Source: CAD feature listing. Evaluate the final solid. Frame: model axes, mm. A direction names the side the tool comes from. Give positions to 0.01 mm unless a question says otherwise; leave off trailing zeros. Write each loop counter-clockwise with the first axis right and the second up, starting at its lowest first coordinate (ties: lowest second). Pieces come first, ordered by that corner, then holes. Notation, with made-up numbers: M -2.75,11 L 14.25,11 A17 ccw 14.25,32 Z; hole C 12,8 d10. An arc over 180 degrees is marked long. Return JSON: item names as keys, results as strings.
Autodesk Inventor part; units mm, degrees
ref_plane "YZ Plane" through (0, 0, 0) normal (1, 0, 0) x (0, 1, 0)
ref_plane "XZ Plane" through (0, 0, 0) normal (0, 1, 0) x (-1, 0, 0)
ref_plane "XY Plane" through (0, 0, 0) normal (0, 0, 1) x (1, 0, 0)
sketch "草图1" plane through (0, 0, 0) normal (0, 1, 0) x (-1, 0, 0)
  line L0 (0, 0) -> (27, 0)
  line L1 (27, 0) -> (27, -44)
  line L2 (27, -44) -> (0, -44)
  line L3 (0, -44) -> (0, 0)
  dimension "d0" = 44
  dimension "d1" = 27
extrude "拉伸1" add sketch "草图1" along normal blind 10
sketch "草图2" plane through (-27, 0, 0) normal (0, 0, 1) x (1, 0, 0)
  line L0 (0, 10) -> (27, 10)
  line L1 (13.5, 10) -> (13.5, 0)
  line L2 (13.5, 10) -> (7.5, 10)
  line L3 (7.5, 10) -> (19.5, 10)
  line L4 (7.5, 10) -> (7.5, 0)
  line L5 (0, 0) -> (27, 0)
  line L6 (19.5, 10) -> (19.5, 0)
  line L7 (7.5, 0) -> (19.5, 0)
  line L8 (7.5, 0) -> (19.5, 0)
  line L9 (19.5, 0) -> (19.5, 8)
  line L10 (19.5, 8) -> (7.5, 8)
  line L11 (7.5, 8) -> (7.5, 0)
  point P0 (7.5, 8)
  dimension "d19" = 6
  dimension "d20" = 12
  dimension "d21" = 8
extrude "拉伸2" cut sketch "草图2" against normal through all contours L10 L1 L5 L4 | L10 L6 L5 L1
sketch "草图3" plane through (-27, 10, 0) normal (0, 0, 1) x (1, 0, 0)
  line L0 (7.5, -10) -> (7.5, -2)
  circle A0 centre (7.5, -6) radius 1.5
  line L1 (19.5, -2) -> (19.5, -10)
  circle A1 centre (19.5, -6) radius 1.5
  point P0 (27, -10)
  point P1 (19.5, -7.5)
  point P2 (19.5, -4.5)
  point P3 (7.5, -4.5)
  point P4 (7.5, -7.5)
  dimension "d22" = 3
  dimension "d23" = 3
extrude "拉伸3" add sketch "草图3" against normal blind 44 contours L0 A0 | L1 A1 picked at (8.2992, -6.2203) picked at (19.2676, -6.4427)
sketch "草图4" plane through (0, 10, 0) normal (0, 1, 0) x (1, 0, 0)
  circle A0 centre (-23, 34) radius 1.5
  line L0 (-6, 44) -> (-21, 44)
  circle A1 centre (-4, 34) radius 1.5
  circle A2 centre (-23, 10) radius 1.5
  circle A3 centre (-4, 10) radius 1.5
  line L1 (-27.606, 22) -> (3.9148, 22)
  line L2 (-13.5, 45.1542) -> (-13.5, -11.9454)
  point P0 (0, 0)
  point P1 (-27, 44)
  dimension "d15" = 3
  dimension "d24" = 12
  dimension "d25" = 9.5
extrude "拉伸4" cut sketch "草图4" against normal blind 10
equation "\"折弯半径\" = 厚度"
equation "\"折弯释压宽度\" = 厚度"
equation "\"折弯释压深度\" = 0.5 * 厚度"
equation "\"拐角释压尺寸\" = 4 * 厚度"
equation "\"最小余量\" = 2 * 厚度"
equation "\"过渡半径\" = 折弯半径"
equation "\"Jacobi半径尺寸\" = 折弯半径"
equation "\"间隙大小\" = 厚度"
properties part number "滑轨座"
1) Draft query along X for faces 4 (the face through (-27, 5, -22)), 5 (the face through (-2.614, 5.07, -9.425)), 6 (the face through (-23.325, 5.07, -32.536)), 7 (the face through (-13.3, 8.3, 0)). Return one class per face: released by +X, released by -X, zero draft, split by the parting line, or undercut.
Numbers:
{"face 4": "released by -X", "face 5": "undercut", "face 6": "undercut", "face 7": "zero draft"}
2) Set-up query: faces 1 (the face through (-18, 4, -22)), 2 (the face through (-24.5, 5.07, -10.07)), 3 (the face through (-7.5, 1, -22)). Return all of +Z, -Z, +X, -X, +Y, -Y with unobstructed straight access to the full face (end or side cutting, diameter ignored); none if empty.
Numbers:
{"face 1": "+Z, -Z", "face 2": "+Y, -Y", "face 3": "+Z, -Z, -Y"}
3) Cut plane A-A, the plane y = 4. Return the cut outline in (x, z), then the cut area to 3 significant figures.
Numbers:
{"outline": "M -27,-44 L -18,-44 L -18,0 L -27,0 Z; M -9,-44 L 0,-44 L 0,0 L -9,0 Z; hole C -23,-34 d3; hole C -23,-10 d3; hole C -4,-34 d3; hole C -4,-10 d3", "area": "764 mm²"}
4) Contact query for flat-ended pins moving along their axis: pin 1 Ø2.5 at (x, z) = (-4, -34) entering from -Y; pin 2 Ø5 at (x, z) = (-15, -37) entering from -Y. Output: stop coordinate, or through.
Numbers:
{"pin 1": "passes through", "pin 2": "stops at y = 8"}
5) Cut plane C-C, the plane z = -10. Return the cut outline in (x, y), then the cut area to 3 significant figures.
Numbers:
{"outline": "M -27,0 L -24.5,0 L -24.5,10 L -27,10 Z; M -21.5,0 L -19.5,0 L -19.5,2.5 A1.5 ccw -19.5,5.5 L -19.5,8 L -7.5,8 L -7.5,5.5 A1.5 ccw -7.5,2.5 L -7.5,0 L -5.5,0 L -5.5,10 L -21.5,10 Z; M -2.5,0 L 0,0 L 0,10 L -2.5,10 Z", "area": "121 mm²"}
6) Cut plane B-B, the plane x = -4. Return the cut outline in (y, z).
Numbers:
{"outline": "M 0,-44 L 10,-44 L 10,-35.5 L 0,-35.5 Z; M 0,-32.5 L 10,-32.5 L 10,-11.5 L 0,-11.5 Z; M 0,-8.5 L 10,-8.5 L 10,0 L 0,0 Z"}
7) Line query: line 1 (Z direction, x = -23, y = 7.25); line 2 (X direction, y = 6.5, z = -10); line 3 (Z direction, x = -22, y = 6.5). Output: solid intervals per line, ascending. Write a range as [from, to].
Numbers:
{"line 1": "z = [-44, -35.5], [-32.5, -11.5], [-8.5, 0]", "line 2": "x = [-27, -24.5], [-21.5, -19.5], [-7.5, -5.5], [-2.5, 0]", "line 3": "z = [-44, -35.12], [-32.88, -11.12], [-8.88, 0]"}
8) Cut plane D-D, the plane y = 9.25. Return the cut outline in (x, z).
Numbers:
{"outline": "M -27,-44 L 0,-44 L 0,0 L -27,0 Z; hole C -23,-34 d3; hole C -23,-10 d3; hole C -4,-34 d3; hole C -4,-10 d3"}
